Geometry check sheet. Reference: drawing and pictorial views, mm from the part's lowest x, y, z. Give positions to 0.01 mm unless a question says otherwise; leave off trailing zeros. Order: outer loops, then holes, each group sorted by start corner. A loop starts at its lowest first (then second) coordinate and runs counter-clockwise, first axis right, second up. Notation, with made-up numbers: (-12, 5) - (19, 5) arc R19 cw to (19, 41) - close; hole circle Ø6 at (53.5, 49.5). An arc over 180 degrees is marked (long way). Answer as a JSON object with one key per item and string values.
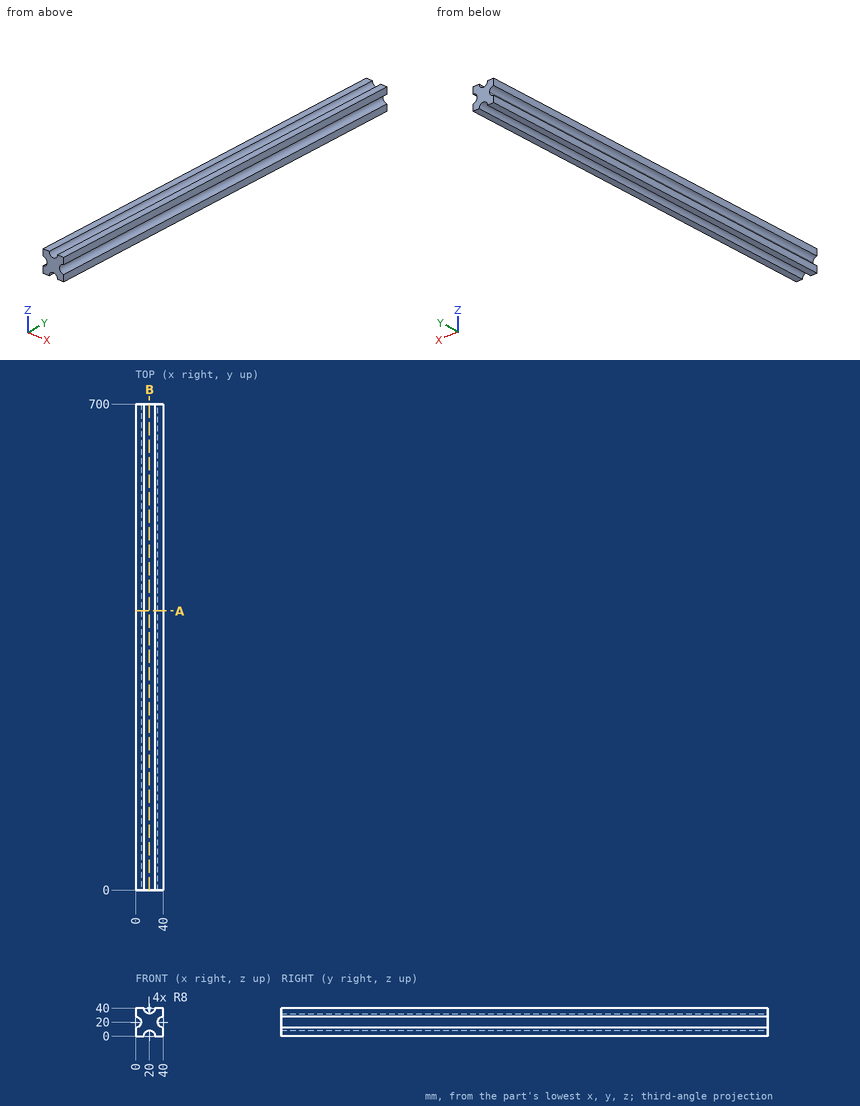
(1) Section check B-B (x = 20). Record the cut outline in (y, z), then the cut area to 3 significant figures.
Computed values:
{"outline": "(0, 8) - (700, 8) - (700, 32) - (0, 32) - close", "area": "16,800 mm²"}
(2) Section check A-A (y = 402). Record the cut outline in (x, z), then the cut area to 3 significant figures.
Computed values:
{"outline": "(0, 0) - (12, 0) arc R8 cw to (28, 0) - (40, 0) - (40, 12) arc R8 cw to (40, 28) - (40, 40) - (28, 40) arc R8 cw to (12, 40) - (0, 40) - (0, 28) arc R8 cw to (8, 20) arc R8 cw to (0, 12) - close", "area": "1,200 mm²"}
(3) Gauge pin test, flat end, axial feed: pin 1 Ø12 at (x, y) = (6, 457.5) entering from -Z. Record the tip position at first contact, or that the pin passes through.
Computed values:
{"pin 1": "stops at z = 0"}
(4) Material ranges on line 1 along Z through (x, y) = (4.5, 153); line 2 along Z through (x, y) = (4, 555), recorded low to high. Write a range as [from, to].
Computed values:
{"line 1": "z = [0, 13.39], [26.61, 40]", "line 2": "z = [0, 13.07], [26.93, 40]"}
